Autodesk Inventor part; units mm, degrees
ref_plane "YZ Plane" through (0, 0, 0) normal (1, 0, 0) x (0, 1, 0)
ref_plane "XZ Plane" through (0, 0, 0) normal (0, 1, 0) x (-1, 0, 0)
ref_plane "XY Plane" through (0, 0, 0) normal (0, 0, 1) x (1, 0, 0)
sketch "Szkic3" plane through (0, 0, 0) normal (0, 1, 0) x (-1, 0, 0)
  circle A0 centre (0, 0) radius 125
  circle A1 centre (0, 0) radius 95
  dimension "d14" = 190
extrude "Wyciągnięcie proste3" add sketch "Szkic3" along normal blind 3
sketch "Szkic4" plane through (0, 0, 0) normal (0, -1, 0) x (1, 0, 0)
  circle A0 centre (0, 0) radius 113
  line L0 (0, 0) -> (0, 141.0619)
  point P0 (20, 111.216)
  point P1 (-20, 111.216)
  point P2 (-106.3159, -38.2875)
  point P3 (-86.3159, -72.9285)
  point P4 (86.3159, -72.9285)
  point P5 (106.3159, -38.2875)
  dimension "d23" = 226
  dimension "d24" = 20
  dimension "d25" = 20
  dimension "d96" = 360
sketch "Szkic7" plane through (0, 0, 0) normal (0, -1, 0) x (1, 0, 0)
  circle A0 centre (0, 0) radius 106.9
  point P0 (106.9, 0)
  point P1 (-53.45, 92.5781)
  point P2 (-53.45, -92.5781)
  dimension "d69" = 213.8
  dimension "d72" = 360
hole "Otwór2" at (106.9, 0, 0) at (-53.45, 0, 92.5781) at (-53.45, 0, -92.5781) direction (0, 1, 0) diameter 4.5 end through all
sketch "Szkic9" plane through (0, 0, 0) normal (0, -1, 0) x (1, 0, 0)
  point P0 (0, 0)
  point P1 (53.45, -92.5781)
  point P2 (53.45, 92.5781)
  point P3 (-106.9, 0)
  dimension "d85" = 360
hole "Otwór3" at (53.45, 0, -92.5781) at (53.45, 0, 92.5781) at (-106.9, 0, 0) direction (0, 1, 0) diameter 3.242 end through all
hole "Otwór4" at (20, 0, 111.216) at (-20, 0, 111.216) at (-106.3159, 0, -38.2875) at (-86.3159, 0, -72.9285) at (86.3159, 0, -72.9285) at (106.3159, 0, -38.2875) direction (0, 1, 0) diameter 3.4 end through all
chamfer "Faza1" distance 0.4 angle 45 9 edges at (86.3159, 0, -71.2285) (106.3159, 0, -36.5875) (-86.3159, 0, -71.2285) (-106.3159, 0, -36.5875) (20, 0, 112.916) (-20, 0, 112.916) (53.45, 3, -90.9571) (-106.9, 3, 1.621) (53.45, 3, 94.1991)
properties part number "RingPrimaryMirror" material "Stal nierdzewna"
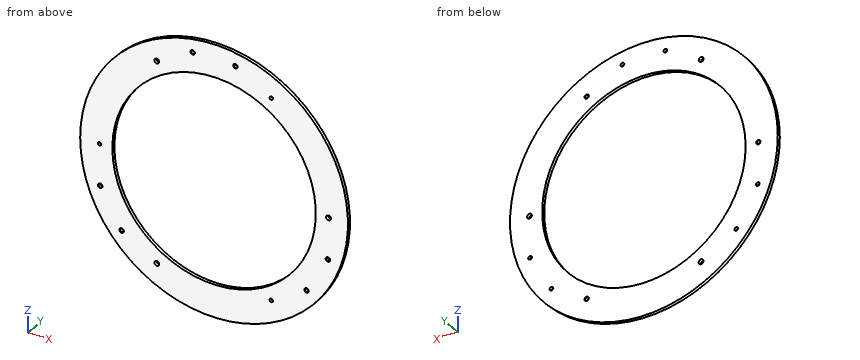
Work out the finished part from the listing and answer in its coordinate system (mm). Round coordinates to 2 decimals unless told otherwise and drop trailing zeros. Write each loop counter-clockwise with the first axis right and the second up, starting at its lowest first coordinate (ties: lowest second). Pieces come first, ordered by that corner, then holes. Notation, with made-up numbers: M 15,86 L 48,86 A34 cw 48,122 Z; hole C -36.75,32 d11. An arc over 180 degrees is marked long. Use a Markdown table: item, result.
1) The part is cut by section D-D on z = -98.5. Give the vertices of the cut face in (x, y), plus the area to 3 significant figures.
Taken from the geometry:
| item | result |
|---|---|
| outline | M -76.96,0 L 76.96,0 L 76.96,3 L -76.96,3 Z |
| area | 462 mm2 |
2) Consider line 1 (Z direction, x = -2.5, y = 2.4) (3 decimals); line 2 (Z direction, x = 19.5, y = 0.7); line 3 (Z direction, x = 106, y = 0.5). Determine where each line is inside the solid, lowest interval first. Write a range as [from, to].
Taken from the geometry:
| item | result |
|---|---|
| line 1 | z = [-124.975, -94.967], [94.967, 124.975] |
| line 2 | z = [-123.47, -92.98], [92.98, 109.59], [112.84, 123.47] |
| line 3 | z = [-66.25, -39.96], [-36.62, -2.06], [2.06, 66.25] |
3) The part is cut by section C-C on y = 1.4. State how many separate pieces and enclosed holes the cut face has, plus the area to 3 significant figures.
Taken from the geometry:
| item | result |
|---|---|
| separate pieces | 1 |
| enclosed holes | 13 |
| area | 20,600 mm2 |
4) The part is cut by section B-B on z = 68. Give the vertices of the cut face in (x, y).
Taken from the geometry:
| item | result |
|---|---|
| outline | M -104.89,0 L -66.34,0 L -66.34,3 L -104.89,3 Z; M 66.34,0 L 104.89,0 L 104.89,3 L 66.34,3 Z |
5) Flat-ended cylindrical pins translate along their axes: pin 1 (1 mm diameter, centred on x = -62.5, y = 1, fed in from +Z); pin 2 (4 mm diameter, centred on x = -86.32, z = -72.93, fed in from -Y); pin 3 (1 mm diameter, centred on x = -98, y = 2, fed in from -Z). Find the tip coordinate at first contact, or state that the pin passes through.
Taken from the geometry:
| item | result |
|---|---|
| pin 1 | stops at z = 108.54 |
| pin 2 | stops at y = 0.1 |
| pin 3 | stops at z = -78.22 |
6) The part is cut by section A-A on x = 0. Give the vertices of the cut face in (y, z).
Taken from the geometry:
| item | result |
|---|---|
| outline | M 0,-125 L 3,-125 L 3,-95 L 0,-95 Z; M 0,95 L 3,95 L 3,125 L 0,125 Z |
